Input: part model. Units: mm. Frame: model coordinates. Give positions to 0.01 mm unless a question says otherwise; leave off trailing zeros. Order: outer loops, then holes, each group sorted by start corner. A loop starts at its lowest first (then second) coordinate and runs counter-clockwise, first axis right, second up. Notation, with made-up numbers: (-15.75, -28) - (-2.75, -28) arc R30 cw to (-2.75, -6) - close; hole circle Ø3 at (-30.5, 85.25). An arc over 180 degrees is marked (long way). Use a Markdown table: item, result.
from build123d import *

# Parameters (mm, degrees)
F0_R     = 11
F0_W     = 80
F0_H     = 30
F1_DEPTH = 6.8
F2_R     = 11
F3_DEPTH = 25
F4_R     = 5


with BuildPart() as f1:
    # F0 (on Top) → F1 (new body)
    with BuildSketch(Plane.XY):
        with Locations((-26, 0)):
            Circle(F0_R)
        with BuildLine():
            ThreePointArc((37, 0), (26, 11), (15, 0))
            ThreePointArc((15, 0), (26, -11), (37, 0))
        make_face()
        with BuildLine():
            ThreePointArc((-11, 0), (0, -11), (11, 0))
            Line((11, 0), (0, 0))
            Line((0, 0), (-11, 0))
        make_face()
        with BuildLine():
            Line((0, 0), (11, 0))
            ThreePointArc((11, 0), (0, 11), (-11, 0))
            Line((-11, 0), (0, 0))
        make_face()
        Rectangle(F0_W, F0_H)
        with Locations((-26, 0)):
            Circle(F0_R, mode=Mode.SUBTRACT)
        with BuildLine():
            ThreePointArc((-11, 0), (0, 11), (11, 0))
            ThreePointArc((11, 0), (0, -11), (-11, 0))
        make_face(mode=Mode.SUBTRACT)
        with BuildLine():
            ThreePointArc((37, 0), (26, -11), (15, 0))
            ThreePointArc((15, 0), (26, 11), (37, 0))
        make_face(mode=Mode.SUBTRACT)
    extrude(amount=F1_DEPTH)

    # F2 (on face) → F3 (cut)
    with BuildSketch(Plane(origin=(0, 0, 0), x_dir=(1, 0, 0), z_dir=(0, 0, -1))):
        with Locations((26, 0)):
            Circle(F2_R)
        Circle(F2_R)
        with Locations((-26, 0)):
            Circle(F2_R)
    extrude(amount=-F3_DEPTH, mode=Mode.SUBTRACT)

    # F4
    f4_edges = [f1.edges().sort_by_distance(p)[0] for p in [
        (-40, -15, 3.4),
        (-40, 15, 3.4),
        (40, 15, 3.4),
        (40, -15, 3.4),
    ]]
    fillet(f4_edges, radius=F4_R)


solid = f1.part
1. Section query A-A (y = 0). Return loops of the section in (x, z), then the cut area to 3 significant figures.
Response:
| item | result |
|---|---|
| outline | (-40, 0) - (-37, 0) - (-37, 6.8) - (-40, 6.8) - close; (-15, 0) - (-11, 0) - (-11, 6.8) - (-15, 6.8) - close; (11, 0) - (15, 0) - (15, 6.8) - (11, 6.8) - close; (37, 0) - (40, 0) - (40, 6.8) - (37, 6.8) - close |
| area | 95.2 mm^2 |
2. Section query B-B (x = -26). Return loops of the section in (y, z), then the cut area to 3 significant figures.
Response:
| item | result |
|---|---|
| outline | (-15, 0) - (-11, 0) - (-11, 6.8) - (-15, 6.8) - close; (11, 0) - (15, 0) - (15, 6.8) - (11, 6.8) - close |
| area | 54.4 mm^2 |
3. Material intervals for line 1 along X through (y, z) = (0.25, 5.5); line 2 along X through (y, z) = (3, 4.75); line 3 along Y through (x, z) = (0, 5.25), sorted ascending.
Response:
| item | result |
|---|---|
| line 1 | x = -40 to -37, -15 to -11, 11 to 15, 37 to 40 |
| line 2 | x = -40 to -36.58, -15.42 to -10.58, 10.58 to 15.42, 36.58 to 40 |
| line 3 | y = -15 to -11, 11 to 15 |
4. Pin query (flat end, axial travel): pin 1 (3 mm diameter, centred on x = -12, y = 10, fed in from -Z). Return the tip coordinate at first contact, or that it passes through.
Response:
| item | result |
|---|---|
| pin 1 | stops at z = 0 |
5. Section query D-D (y = -7). Return loops of the section in (x, z).
Response:
| item | result |
|---|---|
| outline | (-40, 0) - (-34.49, 0) - (-34.49, 6.8) - (-40, 6.8) - close; (-17.51, 0) - (-8.49, 0) - (-8.49, 6.8) - (-17.51, 6.8) - close; (8.49, 0) - (17.51, 0) - (17.51, 6.8) - (8.49, 6.8) - close; (34.49, 0) - (40, 0) - (40, 6.8) - (34.49, 6.8) - close |
6. Mould query, pull axis Y, two halves, no side actions, for faces 1 (the face through (0, -15, 3)), 2 (the face through (-2.38, 10.74, 3.35)), 3 (the face through (39, 13, 3)). Classes: pulls with the +Y half, pulls with the -Y half, needs draft (parallel to the pull), parting line crosses it, or undercut.
Response:
| item | result |
|---|---|
| face 1 | pulls with the -Y half |
| face 2 | undercut |
| face 3 | pulls with the +Y half |
7. Section query C-C (z = 2.5). Return loops of the section in (x, y), then the cut area to 3 significant figures.
Response:
| item | result |
|---|---|
| outline | (-40, -10) arc R5 ccw to (-35, -15) - (35, -15) arc R5 ccw to (40, -10) - (40, 10) arc R5 ccw to (35, 15) - (-35, 15) arc R5 ccw to (-40, 10) - close; hole circle Ø22 at (-26, 0); hole circle Ø22 at (0, 0); hole circle Ø22 at (26, 0) |
| area | 1,240 mm^2 |
